from build123d import *

# Parameters (mm, degrees)
SKIZZE1_R                       = 2.5
AUFSATZ_LINEAR_AUSTRAGEN1_DEPTH = 3.9
VERRUNDUNG1_R                   = 1
FASE1_SIZE                      = 0.25


with BuildPart() as part:
    # Skizze1 → Aufsatz-Linear austragen1 (new body)
    with BuildSketch(Plane.XY):
        Polygon((0, 4.561067127), (3.95, 2.280533563), (3.95, -2.280533563), (0, -4.561067127), (-3.95, -2.280533563), (-3.95, 2.280533563), align=None)
        Circle(SKIZZE1_R, mode=Mode.SUBTRACT)
    extrude(amount=AUFSATZ_LINEAR_AUSTRAGEN1_DEPTH)

    # Verrundung1
    verrundung1_edges = [part.edges().sort_by_distance(p)[0] for p in [
        (0, 4.561067127, 1.95),
        (3.95, 2.280533563, 1.95),
        (3.95, -2.280533563, 1.95),
        (0, -4.561067127, 1.95),
        (-3.95, -2.280533563, 1.95),
        (-3.95, 2.280533563, 1.95),
    ]]
    fillet(verrundung1_edges, radius=VERRUNDUNG1_R)

    # Fase1
    fase1_edges = [part.edges().sort_by_distance(p)[0] for p in [
        (-2.5, 0, 0),
        (-2.5, 0, 3.9),
        (1.975, 3.420800345, 0),
        (1.975, 3.420800345, 3.9),
        (-1.975, 3.420800345, 0),
        (3.95, 0, 0),
        (1.975, -3.420800345, 0),
        (-1.975, -3.420800345, 0),
        (-3.95, 0, 0),
        (0, 4.406366588, 0),
        (-3.816025404, 2.203183294, 0),
        (-3.816025404, -2.203183294, 0),
        (0, -4.406366588, 0),
        (3.816025404, -2.203183294, 0),
        (3.816025404, 2.203183294, 0),
        (3.95, 0, 3.9),
        (-1.975, 3.420800345, 3.9),
        (-3.95, 0, 3.9),
        (-1.975, -3.420800345, 3.9),
        (1.975, -3.420800345, 3.9),
        (0, 4.406366588, 3.9),
        (-3.816025404, 2.203183294, 3.9),
        (-3.816025404, -2.203183294, 3.9),
        (0, -4.406366588, 3.9),
        (3.816025404, -2.203183294, 3.9),
        (3.816025404, 2.203183294, 3.9),
    ]]
    chamfer(fase1_edges, length=FASE1_SIZE)


solid = part.part
Here's how the part is built. I have some questions about the finished solid (model axes, mm). Round coordinates to 2 decimals unless told otherwise and drop trailing zeros. Write each loop counter-clockwise with the first axis right and the second up, starting at its lowest first coordinate (ties: lowest second). Pieces come first, ordered by that corner, then holes. Notation, with made-up numbers: (9.5, -30.5) -> (49.5, -30.5) arc R28 cw to (49.5, 2.5) -> close; hole circle Ø6 at (60, 44.5). An arc over 180 degrees is marked (long way). One line per item, written item: value.
1) We'd pull the mould along X, two halves only. Please class faces 1 (the face through (-1.89, -3.32, 0.12)), 2 (the face through (0.007, 4.406, 1.974)), 3 (the face through (-0.54, -2.44, 1.93)), 4 (the face through (1.996, -3.409, 1.926)): released by +X, released by -X, zero draft, split by the parting line, or undercut.
Filled sheet:
face 1: released by -X
face 2: split by the parting line
face 3: undercut
face 4: released by +X
2) If I drill on line 1 (Y direction, x = 0, z = 1.8); line 2 (Y direction, x = 2, z = 1.45); line 3 (X direction, y = -0.5, z = 2.3), over which ranges is the centre line in solid material (lowest first)? Write a range as [from, to].
Filled sheet:
line 1: y = [-4.41, -2.5], [2.5, 4.41]
line 2: y = [-3.41, -1.5], [1.5, 3.41]
line 3: x = [-3.95, -2.45], [2.45, 3.95]
3) I'm going to push a flat-ended pin straight in: pin 1 Ø1 at (y, z) = (3, 2.5) entering from +X. Where does the tip first touch, or does it pass through?
Filled sheet:
pin 1: stops at x = 3.55
4) Suppose I cut it at D-D on x = 3. List the corners of the cut face in (y, z) for me, plus the area to 3 significant figures.
Filled sheet:
outline: (-2.83, 0.25) -> (-2.54, 0) -> (2.54, 0) -> (2.83, 0.25) -> (2.83, 3.65) -> (2.54, 3.9) -> (-2.54, 3.9) -> (-2.83, 3.65) -> close
area: 21.9 mm2
5) Suppose I cut it at C-C on z = 1.05. List the corners of the cut face in (x, y) for me, plus the area to 3 significant figures.
Filled sheet:
outline: (-3.95, -1.7) arc R1 ccw to (-3.45, -2.57) -> (-0.5, -4.27) arc R1 ccw to (0.5, -4.27) -> (3.45, -2.57) arc R1 ccw to (3.95, -1.7) -> (3.95, 1.7) arc R1 ccw to (3.45, 2.57) -> (0.5, 4.27) arc R1 ccw to (-0.5, 4.27) -> (-3.45, 2.57) arc R1 ccw to (-3.95, 1.7) -> close; hole circle Ø5 at (0, 0)
area: 34.1 mm2
6) Suppose I cut it at A-A on x = 0. List the corners of the cut face in (y, z) for me.
Filled sheet:
outline: (-4.41, 0.25) -> (-4.16, 0) -> (-2.75, 0) -> (-2.5, 0.25) -> (-2.5, 3.65) -> (-2.75, 3.9) -> (-4.16, 3.9) -> (-4.41, 3.65) -> close; (2.5, 0.25) -> (2.75, 0) -> (4.16, 0) -> (4.41, 0.25) -> (4.41, 3.65) -> (4.16, 3.9) -> (2.75, 3.9) -> (2.5, 3.65) -> close
7) Suppose I cut it at B-B on y = 0. List the corners of the cut face in (x, z) for me, plus the area to 3 significant figures.
Filled sheet:
outline: (-3.95, 0.25) -> (-3.7, 0) -> (-2.75, 0) -> (-2.5, 0.25) -> (-2.5, 3.65) -> (-2.75, 3.9) -> (-3.7, 3.9) -> (-3.95, 3.65) -> close; (2.5, 0.25) -> (2.75, 0) -> (3.7, 0) -> (3.95, 0.25) -> (3.95, 3.65) -> (3.7, 3.9) -> (2.75, 3.9) -> (2.5, 3.65) -> close
area: 11.1 mm2
